```python
from build123d import *

# Parameters (mm, degrees)
BOSS_EXTRUDE1_DEPTH = 3
CHAMFER1_SIZE       = 4


with BuildPart() as part:
    # Sketch1 → Boss-Extrude1 (new body)
    with BuildSketch(Plane.XY):
        with BuildLine():
            Line((-21, -21), (21, -21))
            Line((21, -21), (21, 21))
            Line((21, 21), (13.513592999, 28.486407001))
            Line((13.513592999, 28.486407001), (2.845165412, 28.486407001))
            ThreePointArc((2.845165412, 28.486407001), (0, 20.5), (-2.845165412, 28.486407001))
            Line((-2.845165412, 28.486407001), (-13.513592999, 28.486407001))
            Line((-13.513592999, 28.486407001), (-21, 21))
            Line((-21, 21), (-21, -21))
        make_face()
        with BuildLine():
            Line((-11.2, 1.5), (-11.2, -1.5))
            ThreePointArc((-11.2, -1.5), (0, -12.7), (11.2, -1.5))
            Line((11.2, -1.5), (11.2, 1.5))
            ThreePointArc((11.2, 1.5), (0, 12.7), (-11.2, 1.5))
        make_face(mode=Mode.SUBTRACT)
        with BuildLine():
            Line((-13.9, -15), (-13.9, -18))
            ThreePointArc((-13.9, -18), (-15.5, -19.6), (-17.1, -18))
            Line((-17.1, -18), (-17.1, -15))
            ThreePointArc((-17.1, -15), (-15.5, -13.4), (-13.9, -15))
        make_face(mode=Mode.SUBTRACT)
        with BuildLine():
            Line((-13.9, 16), (-13.9, 13))
            ThreePointArc((-13.9, 13), (-15.5, 11.4), (-17.1, 13))
            Line((-17.1, 13), (-17.1, 16))
            ThreePointArc((-17.1, 16), (-15.5, 17.6), (-13.9, 16))
        make_face(mode=Mode.SUBTRACT)
        with BuildLine():
            Line((13.9, -15), (13.9, -18))
            ThreePointArc((13.9, -18), (15.5, -19.6), (17.1, -18))
            Line((17.1, -18), (17.1, -15))
            ThreePointArc((17.1, -15), (15.5, -13.4), (13.9, -15))
        make_face(mode=Mode.SUBTRACT)
        with BuildLine():
            Line((13.9, 16), (13.9, 13))
            ThreePointArc((13.9, 13), (15.5, 11.4), (17.1, 13))
            Line((17.1, 13), (17.1, 16))
            ThreePointArc((17.1, 16), (15.5, 17.6), (13.9, 16))
        make_face(mode=Mode.SUBTRACT)
    extrude(amount=BOSS_EXTRUDE1_DEPTH)

    # Chamfer1
    chamfer1_edges = [part.edges().sort_by_distance(p)[0] for p in [
        (21, -21, 1.5),
        (-21, -21, 1.5),
    ]]
    chamfer(chamfer1_edges, length=CHAMFER1_SIZE)


solid = part.part
```
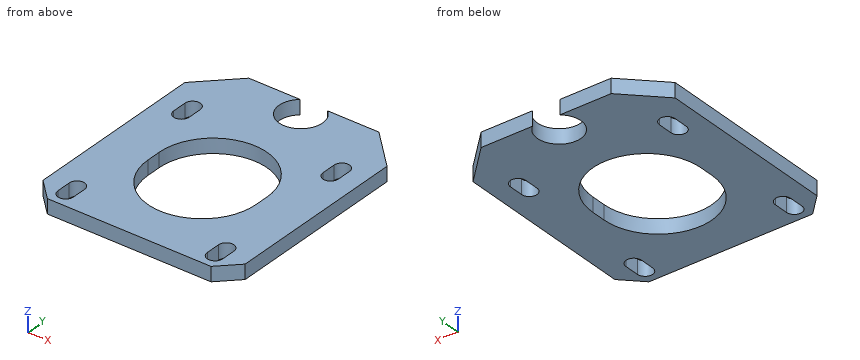
Geometry check sheet. Reference: the model listing, model coordinates, mm. Round coordinates to 2 decimals unless told otherwise and drop trailing zeros. Loops run counter-clockwise (first coordinate to the right, second up) from the corner with the lowest first, then second, coordinate; pieces in that order, holes last. Notation, with made-up numbers: (36.5, 3.5) - (60.5, 3.5) arc R25 ccw to (60.5, 18.5) - close; hole circle Ø3 at (-34.75, -1). An arc over 180 degrees is marked (long way). Write item = value, one per line. Start each with the question number.
1. Depth check by flat-ended pin: pin 1 (8 mm diameter, centred on x = -11, y = -11, fed in from -Z); pin 2 (1 mm diameter, centred on x = -15, z = 1, fed in from +Y). Enter the tip coordinate at first touch or a pass-through.
2. Section check B-B on x = -15.5. Enter the section's corners in (y, z).
3. Section check A-A on y = 25. Enter the section's corners in (x, z), then the cut area to 3 significant figures.
4. Section check D-D on y = -14. Enter the section's corners in (x, z), then the cut area to 3 significant figures.
5. Section check C-C on z = 0.85. Give the number of separate pieces and of enclosed holes in the cut face, then the cut area to 3 significant figures.
6. Thickness scan on line 1 (X direction, y = 25, z = 2.15); line 2 (X direction, y = 1, z = 0.35); line 3 (Y direction, x = -15.5, z = 0.25). Record the ranges inside material, lowest first.
Working result:
q1.pin_1 = 0
q1.pin_2 = 27.5
q2.outline = (-21, 0) - (-19.6, 0) - (-19.6, 3) - (-21, 3) - close; (-13.4, 0) - (11.4, 0) - (11.4, 3) - (-13.4, 3) - close; (17.6, 0) - (26.5, 0) - (26.5, 3) - (17.6, 3) - close
q3.outline = (-17, 0) - (-4.5, 0) - (-4.5, 3) - (-17, 3) - close; (4.5, 0) - (17, 0) - (17, 3) - (4.5, 3) - close
q3.area = 75.0 mm^2
q4.outline = (-21, 0) - (-16.75, 0) - (-16.75, 3) - (-21, 3) - close; (-14.25, 0) - (14.25, 0) - (14.25, 3) - (-14.25, 3) - close; (16.75, 0) - (21, 0) - (21, 3) - (16.75, 3) - close
q4.area = 111 mm^2
q5.separate_pieces = 1
q5.enclosed_holes = 5
q5.area = 1,410 mm^2
q6.line_1 = -17 to -4.5, 4.5 to 17
q6.line_2 = -21 to -11.2, 11.2 to 21
q6.line_3 = -21 to -19.6, -13.4 to 11.4, 17.6 to 26.5
